Autodesk Fusion 360 part; units mm, degrees
sketch "Sketch1" plane through (0, 0, 0) normal (0, 1, 0) x (1, 0, 0)
  line L0 (0, 0) -> (120, 0)
  line L1 (120, 0) -> (120, -60)
  line L2 (120, -60) -> (0, -60)
  line L3 (0, -60) -> (0, 0)
  dimension "d1" = 120
  dimension "d2" = 60
extrude "Extrude1" add sketch "Sketch1" along normal blind 10
sketch "Sketch2" plane through (0, 0, 0) normal (0, -1, 0) x (1, 0, 0)
  line L0 (120, 60) -> (0, 60)
  line L1 (0, 60) -> (0, 0)
  line L2 (0, 0) -> (120, 0)
  line L3 (120, 0) -> (120, 60)
  line L4 (75.5, 45.5) -> (44.5, 45.5)
  line L5 (44.5, 45.5) -> (44.5, 14.5)
  line L6 (44.5, 14.5) -> (75.5, 14.5)
  dimension "d8" = 31
  dimension "d9" = 31
  dimension "d10" = 31
sketch "Sketch3" plane through (0, 0, 0) normal (0, -1, 0) x (1, 0, 0)
  circle A0 centre (44.5, 14.5) radius 1.2645
  circle A1 centre (75.5, 45.5) radius 1.2645
  circle A2 centre (75.5, 14.5) radius 1.2645
  circle A3 centre (44.5, 45.5) radius 1.2645
  line L0 (120, 60) -> (0, 60)
  line L1 (0, 60) -> (0, 0)
  line L2 (0, 0) -> (120, 0)
  line L3 (120, 0) -> (120, 60)
  line L4 (60, 60) -> (60, 30)
  line L5 (120, 60) -> (0, 60)
  line L6 (0, 60) -> (0, 0)
  line L7 (0, 0) -> (120, 0)
  line L8 (120, 0) -> (120, 60)
  dimension "d20" = 30
sketch "Sketch4" plane through (0, 0, 0) normal (0, -1, 0) x (1, 0, 0)
  line L0 (120, 60) -> (0, 60)
  line L1 (0, 60) -> (0, 0)
  line L2 (0, 0) -> (120, 0)
  line L3 (120, 0) -> (120, 60)
sketch "Sketch6" plane through (0, 0, 0) normal (0, -1, 0) x (1, 0, 0)
sketch "Sketch7" plane through (0, 0, 0) normal (0, -1, 0) x (1, 0, 0)
  line L0 (0, 0) -> (60, 0)
  line L1 (60, 0) -> (60, 30)
  line L2 (60, 30) -> (100, 30)
  line L3 (60, 30) -> (20, 30)
  line L4 (20, 30) -> (20, 20)
  line L5 (20, 30) -> (20, 40)
  line L6 (100, 30) -> (100, 20)
  line L7 (100, 30) -> (100, 40)
  dimension "d21" = 60
  dimension "d22" = 30
  dimension "d23" = 40
  dimension "d24" = 40
  dimension "d25" = 10
  dimension "d26" = 10
  dimension "d27" = 10
  dimension "d28" = 10
hole "Hole3" at (60, 0, 30) direction (0, 1, 0) diameter 15.875 depth 25 tip angle 118
sketch "Sketch8" plane through (0, 0, 0) normal (0, -1, 0) x (1, 0, 0)
  line L0 (0, 0) -> (60, 0)
  line L1 (60, 0) -> (60, 30)
  line L2 (60, 30) -> (100, 30)
  line L3 (100, 30) -> (100, 40)
  line L4 (100, 30) -> (100, 20)
  line L5 (100, 40) -> (20, 40)
  line L6 (60, 30) -> (20, 30)
  line L7 (20, 40) -> (20, 20)
  dimension "d32" = 60
  dimension "d33" = 30
  dimension "d34" = 40
  dimension "d35" = 10
  dimension "d36" = 10
  dimension "d37" = 80
  dimension "d38" = 40
  dimension "d39" = 20
hole "Hole4" at (20, 0, 40) at (100, 0, 40) at (100, 0, 20) at (20, 0, 20) direction (0, 1, 0) diameter 4.234 depth 25 tip angle 118
sketch "Sketch9" plane through (0, 0, 0) normal (0, -1, 0) x (1, 0, 0)
  line L0 (70, 40) -> (50, 40)
  line L1 (50, 40) -> (50, 20)
  line L2 (50, 20) -> (70, 20)
  dimension "d47" = 20
  dimension "d48" = 20
  dimension "d49" = 20
hole "Hole5" at (70, 0, 40) at (70, 0, 20) at (50, 0, 40) at (50, 0, 20) direction (0, 1, 0) diameter 2.529 depth 90 tip angle 118
sketch "Sketch5" plane through (0, 0, 0) normal (0, -1, 0) x (1, 0, 0)
The listing builds one solid part. Answer for the finished solid, in the listing's coordinates (mm). Coordinates: 2 decimals unless noted, no trailing zeros. Write each loop counter-clockwise with the first axis right and the second up, starting at its lowest first coordinate (ties: lowest second). Pieces come first, ordered by that corner, then holes.
Q1. Section A-A, the plane z = 20 is taken. Write down the section's boundary in (x, y), then the cut area to 3 significant figures.
Returned:
outline: (0, 0) - (17.88, 0) - (17.88, 10) - (0, 10) - close; (22.12, 0) - (48.74, 0) - (48.74, 10) - (22.12, 10) - close; (51.26, 0) - (68.74, 0) - (68.74, 10) - (51.26, 10) - close; (71.26, 0) - (97.88, 0) - (97.88, 10) - (71.26, 10) - close; (102.12, 0) - (120, 0) - (120, 10) - (102.12, 10) - close
area: 1,060 mm2
Q2. Find the intervals of material crossed by line 1 along X through (y, z) = (7.75, 20); line 2 along Z through (x, y) = (100, 6.25); line 3 along Z through (x, y) = (70, 5.25), in increasing order.
Returned:
line 1: x = 0 to 17.88, 22.12 to 48.74, 51.26 to 68.74, 71.26 to 97.88, 102.12 to 120
line 2: z = 0 to 17.88, 22.12 to 37.88, 42.12 to 60
line 3: z = 0 to 18.74, 21.26 to 38.74, 41.26 to 60
Q3. The mould has two halves that part along Z. Classify faces 1 (the flat face through (0, 5, 30)), 2 (the cylindrical face through (51.234, 5.07, 40.274)), 3 (the flat face through (61, 5, 60)), 4 (the cylindrical face through (68.746, 5.07, 40.165)): released by +Z, released by -Z, zero draft, split by the parting line, or undercut.
Returned:
face 1: zero draft
face 2: undercut
face 3: released by +Z
face 4: undercut
Q4. Section C-C, the plane y = 2.25 is taken. Give the number of separate pieces and of enclosed holes in the cut face, then the cut area to 3 significant figures.
Returned:
separate pieces: 1
enclosed holes: 9
area: 6,930 mm2
Q5. Section B-B, the plane x = 60 is taken. Write down the section's boundary in (y, z).
Returned:
outline: (0, 0) - (10, 0) - (10, 22.06) - (0, 22.06) - close; (0, 37.94) - (10, 37.94) - (10, 60) - (0, 60) - close
Q6. Section D-D, the plane z = 26 is taken. Write down the section's boundary in (x, y).
Returned:
outline: (0, 0) - (53.14, 0) - (53.14, 10) - (0, 10) - close; (66.86, 0) - (120, 0) - (120, 10) - (66.86, 10) - close
